Geometry check sheet. Reference: the model listing, model coordinates, mm. A direction names the side the tool comes from. Round coordinates to 2 decimals unless told otherwise and drop trailing zeros. Order: outer loops, then holes, each group sorted by start corner. A loop starts at its lowest first (then second) coordinate and runs counter-clockwise, first axis right, second up. Notation, with made-up numbers: (41, 3.25) -> (57, 3.25) arc R26 cw to (57, 29.25) -> close; hole circle Ø10 at (81.25, 82). An arc over 180 degrees is marked (long way). Answer as a JSON object with one key per item and string values. Group by question number.
from build123d import *

# Parameters (mm, degrees)
BOSS_EXTRUDE1_DEPTH = 250
BOSS_EXTRUDE2_DEPTH = 25
CUT_EXTRUDE1_DEPTH  = 20
BOSS_EXTRUDE3_DEPTH = 25
CUT_EXTRUDE2_DEPTH  = 20
BOSS_EXTRUDE4_DEPTH = 5
BOSS_EXTRUDE5_DEPTH = 5
SKETCH8_R           = 1.5
CUT_EXTRUDE3_DEPTH  = 10
SKETCH9_W           = 70
SKETCH9_H           = 5.120472302
BOSS_EXTRUDE7_DEPTH = 250
SKETCH11_R          = 3
CUT_EXTRUDE4_DEPTH  = 90


with BuildPart() as part:
    # Sketch1 → Boss-Extrude1 (new body)
    with BuildSketch(Plane(origin=(0, 0, 0), x_dir=(0, 0, -1), z_dir=(1, 0, 0))):
        Polygon((-23.04212536, -5.120472302), (67.5, 35.120472302), (158.04212536, -5.120472302), (158.04212536, -10.240944604), (135, 0), (67.5, 30), (0, 0), (-23.04212536, -10.240944604), align=None)
    extrude(amount=-BOSS_EXTRUDE1_DEPTH)

    # Sketch2 → Boss-Extrude2 (add)
    with BuildSketch(Plane(origin=(0, 0, 0), x_dir=(0, 0, -1), z_dir=(1, 0, 0))):
        Polygon((0, 0), (135, 0), (67.5, 30), align=None)
    extrude(amount=-BOSS_EXTRUDE2_DEPTH)

    # Sketch3 → Cut-Extrude1 (cut)
    with BuildSketch(Plane(origin=(0, 0, 0), x_dir=(0, 0, -1), z_dir=(1, 0, 0))):
        Polygon((0, 0), (135, 0), (67.5, 30), align=None)
    extrude(amount=-CUT_EXTRUDE1_DEPTH, mode=Mode.SUBTRACT)

    # Sketch4 → Boss-Extrude3 (add)
    with BuildSketch(Plane.ZY.offset(250)):
        Polygon((-135, 0), (0, 0), (-67.5, 30), align=None)
    extrude(amount=-BOSS_EXTRUDE3_DEPTH)

    # Sketch5 → Cut-Extrude2 (cut)
    with BuildSketch(Plane.ZY.offset(250)):
        Polygon((-135, 0), (0, 0), (-67.5, 29.582678365), align=None)
    extrude(amount=-CUT_EXTRUDE2_DEPTH, mode=Mode.SUBTRACT)

    # Sketch6 → Boss-Extrude4 (add)
    with BuildSketch(Plane(origin=(0, 0, 0), x_dir=(-1, 0, 0), z_dir=(0, -1, 0))):
        with BuildLine():
            ThreePointArc((233.3, 67.5), (235, 69.2), (236.7, 67.5))
            Line((236.7, 67.5), (240, 67.5))
            ThreePointArc((240, 67.5), (237.071067812, 74.571067812), (230, 77.5))
            Line((230, 77.5), (230, 67.5))
            Line((230, 67.5), (233.3, 67.5))
        make_face()
        with BuildLine():
            Line((240, 67.5), (236.7, 67.5))
            ThreePointArc((236.7, 67.5), (235, 65.8), (233.3, 67.5))
            Line((233.3, 67.5), (230, 67.5))
            Line((230, 67.5), (230, 57.5))
            ThreePointArc((230, 57.5), (237.071067812, 60.428932188), (240, 67.5))
        make_face()
        with BuildLine():
            Line((225, 58.839745962), (225, 76.160254038))
            ThreePointArc((225, 76.160254038), (220, 67.5), (225, 58.839745962))
        make_face()
        with BuildLine():
            Line((230, 67.5), (230, 77.5))
            ThreePointArc((230, 77.5), (227.411809549, 77.159258263), (225, 76.160254038))
            Line((225, 76.160254038), (225, 58.839745962))
            ThreePointArc((225, 58.839745962), (227.411809549, 57.840741737), (230, 57.5))
            Line((230, 57.5), (230, 67.5))
        make_face()
    extrude(amount=-BOSS_EXTRUDE4_DEPTH)

    # Sketch7 → Boss-Extrude5 (add)
    with BuildSketch(Plane(origin=(0, 0, 0), x_dir=(-1, 0, 0), z_dir=(0, -1, 0))):
        with BuildLine():
            Line((20, 57.5), (20, 67.5))
            Line((20, 67.5), (16.7, 67.5))
            ThreePointArc((16.7, 67.5), (15, 65.8), (13.3, 67.5))
            Line((13.3, 67.5), (10, 67.5))
            ThreePointArc((10, 67.5), (12.928932188, 60.428932188), (20, 57.5))
        make_face()
        with BuildLine():
            Line((16.7, 67.5), (20, 67.5))
            Line((20, 67.5), (20, 77.5))
            ThreePointArc((20, 77.5), (12.928932188, 74.571067812), (10, 67.5))
            Line((10, 67.5), (13.3, 67.5))
            ThreePointArc((13.3, 67.5), (15, 69.2), (16.7, 67.5))
        make_face()
        with BuildLine():
            Line((20, 77.5), (20, 67.5))
            Line((20, 67.5), (20, 57.5))
            ThreePointArc((20, 57.5), (22.588190451, 57.840741737), (25, 58.839745962))
            Line((25, 58.839745962), (25, 76.160254038))
            ThreePointArc((25, 76.160254038), (22.588190451, 77.159258263), (20, 77.5))
        make_face()
        with BuildLine():
            ThreePointArc((30, 67.5), (28.660254038, 72.5), (25, 76.160254038))
            Line((25, 76.160254038), (25, 58.839745962))
            ThreePointArc((25, 58.839745962), (28.660254038, 62.5), (30, 67.5))
        make_face()
    extrude(amount=-BOSS_EXTRUDE5_DEPTH)

    # Sketch8 → Cut-Extrude3 (cut)
    with BuildSketch(Plane.ZY.offset(230)):
        with Locations((-67.5, 25)):
            Circle(SKETCH8_R)
    extrude(amount=-CUT_EXTRUDE3_DEPTH, mode=Mode.SUBTRACT)

    # Sketch9 → Boss-Extrude7 (add)
    with BuildSketch(Plane.ZY.offset(250)):
        with Locations((58.04212536, -7.680708453)):
            Rectangle(SKETCH9_W, SKETCH9_H)
    extrude(amount=-BOSS_EXTRUDE7_DEPTH)

    # Sketch11 → Cut-Extrude4 (cut)
    with BuildSketch(Plane(origin=(0, -5.120472302, 0), x_dir=(1, 0, 0), z_dir=(0, 1, 0))):
        with Locations(Location((-225, -70, 0), (0, 0, 270))):
            Circle(SKETCH11_R)
        with Locations(Location((-25, -70, 0), (0, 0, 270))):
            Circle(SKETCH11_R)
    extrude(amount=-CUT_EXTRUDE4_DEPTH, mode=Mode.SUBTRACT)


solid = part.part
Item 1: Sectioned sample at A-A, the plane x = -70.5. Enter the section's corners in (y, z), then the cut area to 3 significant figures.
Item 2: Sectioned sample at B-B, the plane z = -106. Enter the section's corners in (x, y).
Item 3: Set-up check for faces 1 (the flat face through (-127, -5.12, 58)), 2 (the flat face through (-25, 12, -67)), 3 (the flat face through (-17, 5, -68)), 4 (the flat face through (-228, 0, -68)), 5 (the flat face through (-230, 8, -68)): record each of +Z, -Z, +X, -X, +Y, -Y from which the full face is reachable in a straight line by a thin tool's end or side.
Item 4: Depth check by flat-ended pin: pin 1 Ø8 at (x, z) = (-138.5, 56.5) entering from +Y; pin 2 Ø4 at (y, z) = (25, -67.5) entering from +X; pin 3 Ø8 at (x, y) = (-109, 28) entering from -Z. Enter the tip coordinate at first touch or a pass-through.
Item 5: Thickness scan on L1, parallel to X at y = -8, z = 70; L2, parallel to X at y = 1.3, z = -67.5; L3, parallel to X at y = 12, z = -58. Record the ranges inside material, lowest first.
Item 6: Mould release check, pull along X, two halves, no side actions. Record for faces 6 (the flat face through (-240.14, 14.584, -33.278)), 7 (the flat face through (-250, 16, -33)), 8 (the flat face through (-225, 9, -68)): pulls with the +X half, pulls with the -X half, needs draft (parallel to the pull), parting line crosses it, or undercut.
Item 7: Sectioned sample at C-C, the plane z = -16. Enter the section's corners in (x, y), then the cut area to 3 significant figures.
Result:
{
 "1": {"outline": "(-10.24, -158.04) -> (-5.12, -158.04) -> (35.12, -67.5) -> (-5.12, 23.04) -> (-5.12, 93.04) -> (-10.24, 93.04) -> (-10.24, 23.04) -> (30, -67.5) -> close", "area": "1,290 mm2"},
 "2": {"outline": "(-250, 12.71) -> (-230, 12.71) -> (-230, 0) -> (-225, 0) -> (-225, 12.89) -> (-25, 12.89) -> (-25, 0) -> (-20, 0) -> (-20, 12.89) -> (0, 12.89) -> (0, 18.01) -> (-250, 18.01) -> close"},
 "3": {"face 1": "+Z, +X, -X, +Y", "face 2": "none", "face 3": "+X", "face 4": "+X, -X, -Y", "face 5": "-X"},
 "4": {"pin 1": "stops at y = -5.12", "pin 2": "stops at x = -20", "pin 3": "stops at z = -92.52"},
 "5": {"L1": "x = -250 to -228, -222 to -28, -22 to 0", "L2": "x = -240 to -236.7, -233.3 to -220, -30 to -16.7, -13.3 to -10", "L3": "x = -230 to -225, -25 to -20"},
 "6": {"face 6": "needs draft", "face 7": "pulls with the -X half", "face 8": "undercut"},
 "7": {"outline": "(-250, 7.01) -> (-230, 7.01) -> (-230, 0) -> (-225, 0) -> (-225, 7.11) -> (-25, 7.11) -> (-25, 0) -> (-20, 0) -> (-20, 7.11) -> (0, 7.11) -> (0, 12.23) -> (-250, 12.23) -> close", "area": "1,350 mm2"}
}
